Build history of the part. All positions in model axes, mm. A direction names the side the tool comes from. Round coordinates to 2 decimals unless told otherwise and drop trailing zeros. Loops run counter-clockwise (first coordinate to the right, second up) from the corner with the lowest first, then second, coordinate; pieces in that order, holes last. Notation, with made-up numbers: (49.5, -28) - (86.5, -28) arc R12 ccw to (86.5, -9) - close; hole circle Ø3 at (33.5, 30.25). An arc over 180 degrees is marked (long way). Answer as CSV lines item,"result". Start each with the question number.
```python
from build123d import *

# Parameters (mm, degrees)
IZIM2_W                          = 40
IZIM2_H                          = 16
Y_KSEKLIK_EKSTR_ZYON4_DEPTH      = 9
Y_KSEKLIK_EKSTR_ZYON5_DEPTH      = 2
Y_KSEKLIK_EKSTR_ZYON5_DEPTH_BACK = 42
Y_KSEKLIK_EKSTR_ZYON6_DEPTH      = 6
Y_KSEKLIK_EKSTR_ZYON6_DEPTH_BACK = 46
KES_EKSTR_ZYON1_DEPTH            = 52
KES_EKSTR_ZYON2_DEPTH            = 53.347615077
KES_EKSTR_ZYON2_DEPTH_BACK       = 52
IZIM3_4_W                        = 9
IZIM3_4_H                        = 16
Y_KSEKLIK_EKSTR_ZYON7_DEPTH      = 44
KES_EKSTR_ZYON4_DEPTH            = 44
KES_EKSTR_ZYON8_DEPTH            = 2.2
KES_EKSTR_ZYON9_DEPTH            = 2.2
IZIM14_W                         = 39.6
IZIM14_H                         = 3
ARALIK_EKS_DEPTH                 = 0.6
Y_KSEKLIK_EKSTR_ZYON9_DEPTH      = 12
Y_KSEKLIK_EKSTR_ZYON10_DEPTH     = 50
IZIM17_R                         = 1.95
IZIM17_W                         = 4.9
IZIM17_H                         = 4.9
Y_KSEKLIK_EKSTR_ZYON11_DEPTH     = 3.4
KES_EKSTR_ZYON11_DEPTH           = 0.8
KES_EKSTR_ZYON12_DEPTH           = 2


with BuildPart() as part:
    # izim2 → Y_kseklik-Ekstr_zyon4 (new body)
    with BuildSketch(Plane.XY):
        with Locations((-27.243761407, 15.308213235)):
            Rectangle(IZIM2_W, IZIM2_H)
    extrude(amount=Y_KSEKLIK_EKSTR_ZYON4_DEPTH)

    # izim3 → Y_kseklik-Ekstr_zyon5 (add, two sides: drawn at the far end of the back side and taken through both)
    with BuildSketch(Plane(origin=(-7.243761407, 0, 0), x_dir=(0, 0, -1), z_dir=(1, 0, 0)).offset(-Y_KSEKLIK_EKSTR_ZYON5_DEPTH_BACK)):
        with BuildLine():
            ThreePointArc((-9, 9.308213235), (-3, 15.308213235), (-9, 21.308213235))
            Line((-9, 21.308213235), (-9, 19.308213235))
            ThreePointArc((-9, 19.308213235), (-5, 15.308213235), (-9, 11.308213235))
            Line((-9, 11.308213235), (-9, 9.308213235))
        make_face()
    extrude(amount=Y_KSEKLIK_EKSTR_ZYON5_DEPTH + Y_KSEKLIK_EKSTR_ZYON5_DEPTH_BACK)

    # izim3_3 → Y_kseklik-Ekstr_zyon6 (add, two sides: drawn at the far end of the back side and taken through both)
    with BuildSketch(Plane(origin=(-7.243761407, 0, 0), x_dir=(0, 0, -1), z_dir=(1, 0, 0)).offset(-Y_KSEKLIK_EKSTR_ZYON6_DEPTH_BACK)):
        with BuildLine():
            ThreePointArc((-9, 11.308213235), (-5, 15.308213235), (-9, 19.308213235))
            Line((-9, 19.308213235), (-9, 11.308213235))
        make_face()
    extrude(amount=Y_KSEKLIK_EKSTR_ZYON6_DEPTH + Y_KSEKLIK_EKSTR_ZYON6_DEPTH_BACK)

    # izim4 → Kes-Ekstr_zyon1 (cut)
    with BuildSketch(Plane(origin=(-1.243761407, 0, 0), x_dir=(0, 0, -1), z_dir=(1, 0, 0))):
        with BuildLine():
            Line((-9, 17.308213235), (-9, 13.308213235))
            ThreePointArc((-9, 13.308213235), (-7, 15.308213235), (-9, 17.308213235))
        make_face()
    extrude(amount=-KES_EKSTR_ZYON1_DEPTH, mode=Mode.SUBTRACT)

    # izim3_4 → Kes-Ekstr_zyon2 (cut, two sides: drawn at the far end of the back side and taken through both)
    with BuildSketch(Plane(origin=(-7.243761407, 0, 0), x_dir=(0, 0, -1), z_dir=(1, 0, 0)).offset(-KES_EKSTR_ZYON2_DEPTH_BACK)):
        with Locations((-4.5, 15.308213235)):
            Rectangle(IZIM3_4_W, IZIM3_4_H)
        with BuildLine():
            ThreePointArc((-9, 9.308213235), (-3, 15.308213235), (-9, 21.308213235))
            Line((-9, 21.308213235), (-9, 9.308213235))
        make_face(mode=Mode.SUBTRACT)
    extrude(amount=KES_EKSTR_ZYON2_DEPTH + KES_EKSTR_ZYON2_DEPTH_BACK, mode=Mode.SUBTRACT)


with BuildPart() as kes_ekstr_zyon2_kept_piece:
    # of the separate pieces the step leaves, the one the design keeps (kes_ekstr_zyon2_pieces_kept)
    add(part.part.solids().sort_by_distance((-49.243761407, 9.308213235, 9))[0])

    # izim7 → Y_kseklik-Ekstr_zyon7 (add)
    with BuildSketch(Plane(origin=(-5.243761407, 0, 0), x_dir=(0, 0, -1), z_dir=(1, 0, 0))):
        with BuildLine():
            Line((-5, 19.78034919), (-5, 24.308213235))
            Line((-5, 24.308213235), (-9, 24.308213235))
            Line((-9, 24.308213235), (-9, 21.308213235))
            ThreePointArc((-9, 21.308213235), (-6.859067461, 20.913247389), (-5, 19.78034919))
        make_face()
    extrude(amount=-Y_KSEKLIK_EKSTR_ZYON7_DEPTH)

    # izim8 → Kes-Ekstr_zyon4 (cut)
    with BuildSketch(Plane.XY.offset(9)):
        Polygon((-7.443761407, 24.308213235), (-7.443761407, 21.308213235), (-5.243761407, 21.308213235), (-5.243761407, 22.308213235), (-5.243761407, 24.308213235), align=None)
        Polygon((-49.243761407, 24.308213235), (-47.043761407, 24.308213235), (-47.043761407, 21.308213235), (-49.243761407, 21.308213235), (-49.243761407, 22.308213235), align=None)
    extrude(amount=-KES_EKSTR_ZYON4_DEPTH, mode=Mode.SUBTRACT)

    # izim7_3 → Kes-Ekstr_zyon8 (cut)
    with BuildSketch(Plane(origin=(-5.243761407, 0, 0), x_dir=(0, 0, -1), z_dir=(1, 0, 0))):
        with BuildLine():
            Line((-5, 19.78034919), (-5, 24.308213235))
            Line((-5, 24.308213235), (-9, 24.308213235))
            Line((-9, 24.308213235), (-9, 21.308213235))
            ThreePointArc((-9, 21.308213235), (-6.859067461, 20.913247389), (-5, 19.78034919))
        make_face()
    extrude(amount=-KES_EKSTR_ZYON8_DEPTH, mode=Mode.SUBTRACT)

    # izim12 → Kes-Ekstr_zyon9 (cut)
    with BuildSketch(Plane.ZY.offset(49.243761407)):
        with BuildLine():
            Line((5, 19.78034919), (5, 21.308213235))
            Line((5, 21.308213235), (9, 21.308213235))
            ThreePointArc((9, 21.308213235), (6.859067461, 20.913247389), (5, 19.78034919))
        make_face()
    extrude(amount=-KES_EKSTR_ZYON9_DEPTH, mode=Mode.SUBTRACT)

    # izim14 → aralik_eks (add)
    with BuildSketch(Plane(origin=(0, 24.308213235, 0), x_dir=(1, 0, 0), z_dir=(0, 1, 0))):
        with Locations((-27.243761407, -7.5)):
            Rectangle(IZIM14_W, IZIM14_H)
    extrude(amount=ARALIK_EKS_DEPTH)

    # izim15 → Y_kseklik-Ekstr_zyon9 (add)
    with BuildSketch(Plane(origin=(0, 24.908213235, 0), x_dir=(1, 0, 0), z_dir=(0, 1, 0))):
        Polygon((-47.043761407, -6), (-67.043761407, -6), (-67.043761407, -9), (-47.043761407, -9), (-7.443761407, -9), (12.556238593, -9), (12.556238593, -6), (-7.443761407, -6), align=None)
    extrude(amount=Y_KSEKLIK_EKSTR_ZYON9_DEPTH)

    # izim16 → Y_kseklik-Ekstr_zyon10 (add)
    with BuildSketch(Plane.XY.offset(9)):
        Polygon((-67.043761407, 36.908213235), (12.556238593, 36.908213235), (12.556238593, 31.908213235), (9.556238593, 31.908213235), (9.556238593, 35.308213235), (-64.043761407, 35.308213235), (-64.043761407, 31.908213235), (-67.043761407, 31.908213235), align=None)
    extrude(amount=Y_KSEKLIK_EKSTR_ZYON10_DEPTH)

    # izim17 → Y_kseklik-Ekstr_zyon11 (add)
    # profile 1 of 3: a face of its own
    with BuildSketch(Plane.XZ.offset(-35.308213235)):
        Polygon((9.556238593, 59), (-64.043761407, 59), (-64.043761407, 51.1), (-59.143761407, 51.1), (-59.143761407, 56), (4.656238593, 56), (4.656238593, 51.1), (9.556238593, 51.1), align=None)
        with Locations(Location((-61.593761407, 53.55, 0), (0, 0, 270))):
            Circle(IZIM17_R, mode=Mode.SUBTRACT)
        with Locations(Location((7.106238593, 53.55, 0), (0, 0, 270))):
            Circle(IZIM17_R, mode=Mode.SUBTRACT)
    # profile 2 of 3: a face of its own
    with BuildSketch(Plane.XZ.offset(-35.308213235)):
        with Locations((7.106238593, 14.45)):
            Rectangle(IZIM17_W, IZIM17_H)
        with Locations(Location((7.106238593, 14.45, 0), (0, 0, 90))):
            Circle(IZIM17_R, mode=Mode.SUBTRACT)
    # profile 3 of 3: a face of its own
    with BuildSketch(Plane.XZ.offset(-35.308213235)):
        with Locations((-61.593761407, 14.45)):
            Rectangle(IZIM17_W, IZIM17_H)
        with Locations(Location((-61.593761407, 14.45, 0), (0, 0, 90))):
            Circle(IZIM17_R, mode=Mode.SUBTRACT)
    extrude(amount=Y_KSEKLIK_EKSTR_ZYON11_DEPTH)

    # izim18 → Kes-Ekstr_zyon11 (cut)
    with BuildSketch(Plane.XY.offset(9)):
        with BuildLine():
            Line((-39.543761407, 28.308213235), (-39.543761407, 17.308213235))
            ThreePointArc((-39.543761407, 17.308213235), (-38.000834326, 15.938341904), (-36.30655982, 14.760799827))
            Line((-36.30655982, 14.760799827), (-18.180962994, 14.760799827))
            ThreePointArc((-18.180962994, 14.760799827), (-16.486688488, 15.938341904), (-14.943761407, 17.308213235))
            Line((-14.943761407, 17.308213235), (-14.943761407, 28.308213235))
            Line((-14.943761407, 28.308213235), (-7.443761407, 35.308213235))
            Line((-7.443761407, 35.308213235), (-47.043761407, 35.308213235))
            Line((-47.043761407, 35.308213235), (-39.543761407, 28.308213235))
        make_face()
    extrude(amount=-KES_EKSTR_ZYON11_DEPTH, mode=Mode.SUBTRACT)

    # izim19 → Kes-Ekstr_zyon12 (cut)
    with BuildSketch(Plane.XY.offset(9)):
        Polygon((-10.243761407, 18.606911619), (-8.625727418, 19.782482123), (-9.243761407, 21.684595156), (-11.243761407, 21.684595156), (-11.861795396, 19.782482123), align=None)
        Polygon((-42.625727418, 19.782482123), (-44.243761407, 18.606911619), (-45.861795396, 19.782482123), (-45.243761407, 21.684595156), (-43.243761407, 21.684595156), align=None)
    extrude(amount=-KES_EKSTR_ZYON12_DEPTH, mode=Mode.SUBTRACT)


solid = kes_ekstr_zyon2_kept_piece.part
```
Q1. Pin check, flat tips, straight feed: pin 1 Ø3.5 at (x, y) = (-61, 33) entering from -Z; pin 2 Ø2.5 at (x, z) = (-61.59, 53.55) entering from -Y; pin 3 Ø1.5 at (x, y) = (-43.5, 20) entering from +Z. Stop position of each tip, or through.
Q2. Band-saw the part on A-A, the plane z = 14.45. List the corners of the cut face in (x, y).
Q3. Two-plate mould, pull along Y, no slides. Class faces 6 (the flat face through (-57, 24.908, 7)), 7 (the flat face through (7, 35.308, 54)), 8 (the flat face through (-9.446, 19.186, 8.014)), 9 (the flat face through (-62, 34, 51.1)): released by +Y, released by -Y, zero draft, split by the parting line, or undercut.
Q4. Band-saw the part on B-B, the plane x = -57. List the corners of the cut face in (y, z), then the cut area to 3 significant figures.
Q5. Tool access for faces 1 (the flat face through (-10, 20, 7)), 2 (the flat face through (-5.244, 15.4, 4.7)), 3 (the flat face through (9.556, 34, 34)), 4 (the flat face through (-67.044, 33, 32)), 5 (the flat face through (-49.244, 15.4, 4.7)): list every direction of +Z, -Z, +X, -X, +Y, -Y with a clear straight run to the whole face (end or side of a thin tool).
Q6. Wall check: probe 1 along X at (y, z) = (33.5, 53.5); probe 2 along X at (y, z) = (34, 29.5); probe 3 along Z at (x, y) = (-10.5, 33). Give the ranges that are in metal, low to high. Write a range as [from, to].
Q7. Band-saw the part on D-D, the plane y = 33. List the corners of the cut face in (x, z), then the cut area to 3 significant figures.
Q8. Band-saw the part on C-C, the plane y = 15.75. List the corners of the cut face in (x, z), then the cut area to 3 significant figures.
Reported:
1,pin 1,"stops at z = 6"
1,pin 2,"stops at y = 35.31"
1,pin 3,"stops at z = 9"
2,outline,"(-67.04, 31.91) - (-63.54, 31.91) - (-63.54, 35.31) - (-59.64, 35.31) - (-59.64, 31.91) - (-59.14, 31.91) - (-59.14, 35.31) - (4.66, 35.31) - (4.66, 31.91) - (5.16, 31.91) - (5.16, 35.31) - (9.06, 35.31) - (9.06, 31.91) - (12.56, 31.91) - (12.56, 36.91) - (-67.04, 36.91) - close"
3,face 6,"undercut"
3,face 7,"released by -Y"
3,face 8,"undercut"
3,face 9,"zero draft"
4,outline,"(24.91, 6) - (36.91, 6) - (36.91, 59) - (31.91, 59) - (31.91, 56) - (35.31, 56) - (35.31, 9) - (24.91, 9) - close"
4,area,"126 mm2"
5,face 1,"+Z"
5,face 2,"-Z, +X"
5,face 3,"-Y"
5,face 4,"+Z, -Z, -X, +Y, -Y"
5,face 5,"-Z, -X"
6,probe 1,"x = [-67.04, -63.54], [-59.64, -59.14], [4.66, 5.16], [9.06, 12.56]"
6,probe 2,"x = [-67.04, -64.04], [9.56, 12.56]"
6,probe 3,"z = [6, 8.2], [56, 59]"
7,outline,"(-67.04, 6) - (12.56, 6) - (12.56, 59) - (-67.04, 59) - close; hole (-64.04, 9) - (-44.57, 9) - (-44.57, 8.2) - (-9.92, 8.2) - (-9.92, 9) - (9.56, 9) - (9.56, 12) - (4.66, 12) - (4.66, 16.9) - (9.56, 16.9) - (9.56, 51.1) - (4.66, 51.1) - (4.66, 56) - (-59.14, 56) - (-59.14, 51.1) - (-64.04, 51.1) - (-64.04, 16.9) - (-59.14, 16.9) - (-59.14, 12) - (-64.04, 12) - close; hole circle Ø3.9 at (-61.59, 14.45); hole circle Ø3.9 at (-61.59, 53.55); hole circle Ø3.9 at (7.11, 14.45); hole circle Ø3.9 at (7.11, 53.55)"
7,area,"780 mm2"
8,outline,"(-53.24, 5.02) - (-49.24, 5.02) - (-49.24, 3.02) - (-5.24, 3.02) - (-5.24, 5.02) - (-1.24, 5.02) - (-1.24, 7.05) - (-53.24, 7.05) - close"
8,area,"194 mm2"
